Input: dimensioned drawing with shaded views. Units: mm. Origin: part minimum x, y, z. A direction names the side the tool comes from. Give positions to 0.01 mm unless a question says otherwise; leave off trailing zeros. Write each loop counter-clockwise with the first axis right and the second up, starting at its lowest first coordinate (ties: lowest second). Pieces come first, ordered by that corner, then holes. Notation, with made-up numbers: M -18.5,5 L 21.5,5 A27 cw 21.5,25 Z; hole C -21.5,-11.5 d3. An arc over 180 degrees is marked long. Answer as a JSON object with one key per item and string values.
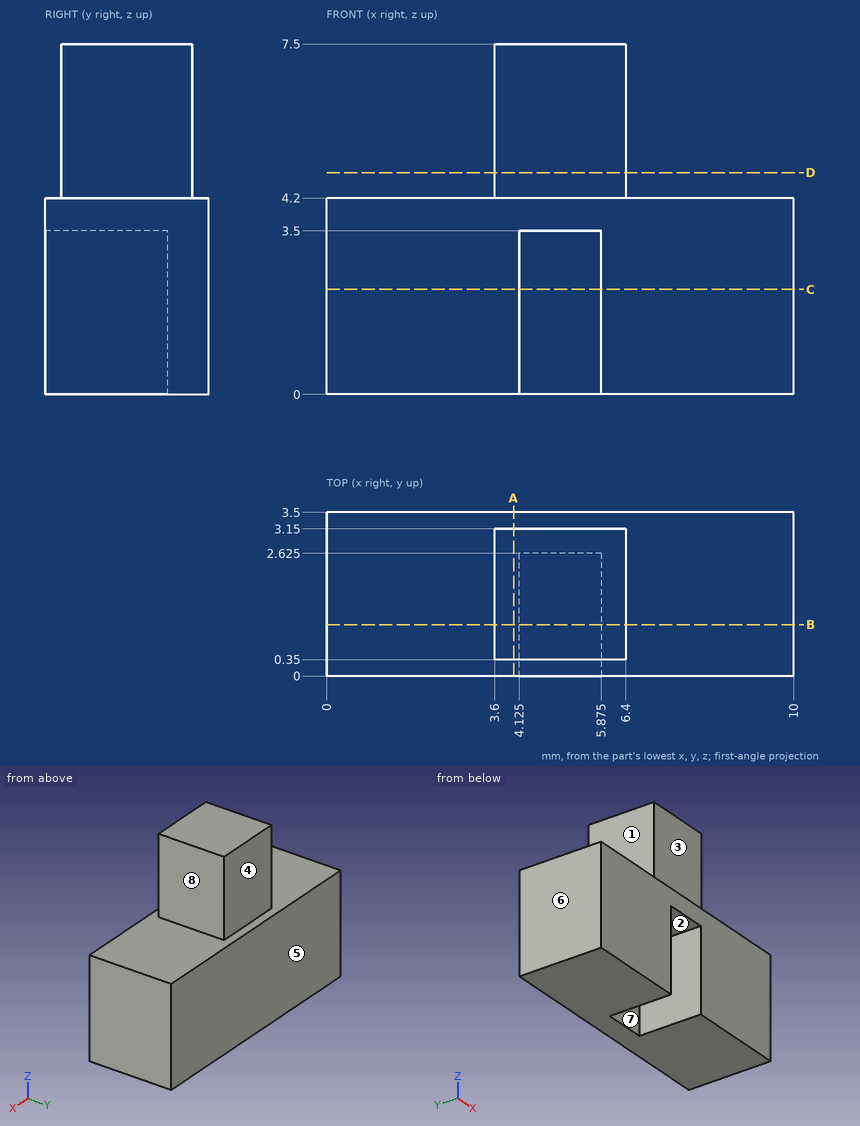
1) Line query: line 1 (X direction, y = 1.95, z = 2.25) (3 decimals); line 2 (Z direction, x = 5, y = 2.2); line 3 (X direction, y = 0.4, z = 4.75). Output: solid intervals per line, ascending. Write a range as from..to.
Geometry check:
{"line 1": "x = 0..4.125, 5.875..10", "line 2": "z = 3.5..7.5", "line 3": "x = 3.6..6.4"}
2) Set-up query: the marked faces 1, 2, 3 and 4. Return all of +Z, -Z, +X, -X, +Y, -Y with unobstructed straight access to the full face (end or side cutting, diameter ignored); none if empty.
Geometry check:
{"face 1": "+Z, -X, +Y, -Y", "face 2": "-Z, -Y", "face 3": "+Z, +X, -X, -Y", "face 4": "+Z, +X, -X, +Y"}
3) Cut plane A-A on x = 4. Return loops of the section in (y, z), and give its area (3 significant figures).
Geometry check:
{"outline": "M 0,0 L 3.5,0 L 3.5,4.2 L 3.15,4.2 L 3.15,7.5 L 0.35,7.5 L 0.35,4.2 L 0,4.2 Z", "area": "23.9 mm2"}
4) Cut plane C-C on z = 2.25. Return loops of the section in (x, y) (3 decimals), and give its area (3 significant figures).
Geometry check:
{"outline": "M 0,0 L 4.125,0 L 4.125,2.625 L 5.875,2.625 L 5.875,0 L 10,0 L 10,3.5 L 0,3.5 Z", "area": "30.4 mm2"}
5) Pull-direction query (X, two-part tool) for the marked faces 5, 6, 7 and 8; classes: pulls with the +X half, pulls with the -X half, needs draft (parallel to the pull), parting line crosses it, or undercut.
Geometry check:
{"face 5": "needs draft", "face 6": "pulls with the -X half", "face 7": "undercut", "face 8": "pulls with the +X half"}
6) Cut plane D-D on z = 4.75. Return loops of the section in (x, y), and give its area (3 significant figures).
Geometry check:
{"outline": "M 3.6,0.35 L 6.4,0.35 L 6.4,3.15 L 3.6,3.15 Z", "area": "7.84 mm2"}
7) Contact query for flat-ended pins moving along their axis: P1, Ø2, axis at x = 4.5, z = 5.5, coming from the +Y side; P2, Ø0.8, axis at y = 1, z = 6.5, coming from the +X side; P3, Ø2, axis at x = 5.5, z = 6.5, coming from the -Y side. Output: stop coordinate, or through.
Geometry check:
{"P1": "stops at y = 3.15", "P2": "stops at x = 6.4", "P3": "stops at y = 0.35"}
8) Cut plane B-B on y = 1.1. Return loops of the section in (x, z) (3 decimals), and give its area (3 significant figures).
Geometry check:
{"outline": "M 0,0 L 4.125,0 L 4.125,3.5 L 5.875,3.5 L 5.875,0 L 10,0 L 10,4.2 L 6.4,4.2 L 6.4,7.5 L 3.6,7.5 L 3.6,4.2 L 0,4.2 Z", "area": "45.1 mm2"}
